Input: part model. Units: mm. Frame: model coordinates. A direction names the side the tool comes from. Give positions to 0.01 mm unless a question says otherwise; leave off trailing zeros. Order: outer loops, then holes, each group sorted by start corner. A loop starts at its lowest first (then second) coordinate and runs counter-clockwise, first axis right, second up. Notation, with made-up numbers: (-36.5, -12.5) -> (-28.5, -12.5) arc R14 ccw to (-28.5, 13.5) -> close; hole circle Ø7 at (-25.5, 73.25). An arc over 180 degrees is marked (long way). Use a Markdown table: item, result. Add a question column.
Autodesk Inventor part; units mm, degrees
ref_plane "YZ Plane" through (0, 0, 0) normal (1, 0, 0) x (0, 1, 0)
ref_plane "XZ Plane" through (0, 0, 0) normal (0, 1, 0) x (-1, 0, 0)
ref_plane "XY Plane" through (0, 0, 0) normal (0, 0, 1) x (1, 0, 0)
sketch "Sketch1" plane through (0, 0, 0) normal (0, 0, 1) x (1, 0, 0)
  circle A0 centre (0, 0) radius 100
  dimension "d0" = 200
extrude "Extrusion2" add sketch "Sketch1" along normal blind 3
ref_plane "Work Plane1" through (-33, -35, 0) normal (-1, 0, 0) x (0, 0, 1)
sketch "Sketch33" plane through (0, 0, 0) normal (0, 0, -1) x (-1, 0, 0)
  line L0 (-60, 40) -> (-78, 40)
  line L1 (-78, 40) -> (-78, 46)
  line L2 (-78, 46) -> (-60, 46)
  line L3 (-60, 46) -> (-60, 40)
  point P0 (0, 0)
  dimension "d123" = 18
  dimension "d124" = 6
extrude "Extrusion32" cut sketch "Sketch33" against normal blind 1
mirror "Mirror21" about plane through (0, 0, 0) normal (1, 0, 0) of "Extrusion32"
mirror "Mirror22" about plane through (0, 0, 0) normal (0, 1, 0) of "Extrusion32", "Mirror21"
sketch "Sketch34" plane through (0, 0, 1) normal (0, 0, -1) x (-1, 0, 0)
  circle A0 centre (-75, 43) radius 1.5
  circle A1 centre (-63, 43) radius 1.5
  point P0 (0, 0)
  dimension "d127" = 3
  dimension "d128" = 3
extrude "Extrusion33" cut sketch "Sketch34" against normal up to next
mirror "Mirror23" about plane through (0, 0, 0) normal (1, 0, 0) of "Extrusion33"
mirror "Mirror24" about plane through (0, 0, 0) normal (0, 1, 0) of "Extrusion33", "Mirror23"
properties part number "second floor"
Q1. Section query C-C (x = 22). Return loops of the section in (y, z), plus the area to 3 significant figures.
Q2. Section query A-A (z = 2.35). Give the number of separate pieces and of enclosed holes in the cut face, plus the area to 3 significant figures.
Q3. Section query B-B (y = 65.5). Return loops of the section in (x, z).
Q4. Access query for faces 4 (the flat face through (-69, 43, 1)), 5 (the flat face through (-1, 1, 3)). Directions: +Z, -Z, +X, -X, +Y, -Y. A direction counts if a zero-diameter tool reaches every point of the face in a straight line with its end or side. Return the directions, or none.
Q5. Draft query along X for faces 1 (the cylindrical face through (95.38, -30.04, 1.48)), 2 (the flat face through (-1, 1, 0)), 3 (the flat face through (69, -43, 1)). Return one class per face: +X half, -X half, draft (parallel to the pull), parting line (faces both ways), or undercut.
Q6. First-contact query: pin 1 (0.5 mm diameter, centred on x = -71.5, z = 0.5, fed in from +Y); pin 2 (0.8 mm diameter, centred on x = -69, z = 0.5, fed in from -Y); pin 3 (1 mm diameter, centred on x = -4, z = 0.5, fed in from +Y); pin 4 (2.5 mm diameter, centred on x = -63, y = 43, fed in from +Z). Flat tips, straight axial feed; report the tip coordinate or a pass-through.
Q7. Ray query, line 1 (Y direction, x = 76, z = 0.95); line 2 (Y direction, x = -63, z = 1.6); line 3 (X direction, y = 90, z = 1.35). Return the intervals inside material, ascending.
Solution:
| question | item | result |
|---|---|---|
| 1 | outline | (-97.55, 0) -> (97.55, 0) -> (97.55, 3) -> (-97.55, 3) -> close |
| 1 | area | 585 mm² |
| 2 | separate pieces | 1 |
| 2 | enclosed holes | 8 |
| 2 | area | 31,400 mm² |
| 3 | outline | (-75.56, 0) -> (75.56, 0) -> (75.56, 3) -> (-75.56, 3) -> close |
| 4 | face 4 | -Z |
| 4 | face 5 | +Z, +X, -X, +Y, -Y |
| 5 | face 1 | parting line |
| 5 | face 2 | draft |
| 5 | face 3 | undercut |
| 6 | pin 1 | stops at y = 70.17 |
| 6 | pin 2 | stops at y = -72.76 |
| 6 | pin 3 | stops at y = 99.94 |
| 6 | pin 4 | passes through |
| 7 | line 1 | y = -64.99 to -46, -40 to 40, 46 to 64.99 |
| 7 | line 2 | y = -77.66 to -44.5, -41.5 to 41.5, 44.5 to 77.66 |
| 7 | line 3 | x = -43.59 to 43.59 |
